```python
from build123d import *

# Parameters (mm, degrees)
F1_DEPTH = 15
F2_R     = 7.5
F3_DEPTH = 107.336067
F4_R     = 10
F5_DEPTH = 70


with BuildPart() as f1:
    # F0 (on Front) → F1 (new body, symmetric)
    with BuildSketch(Plane.XZ):
        with BuildLine():
            ThreePointArc((-30, 0), (-27.716386, 11.480503), (-21.213203, 21.213203))
            Line((-21.213203, 21.213203), (-70.710678, 70.710678))
            ThreePointArc((-70.710678, 70.710678), (-92.387953, 38.268343), (-100, 0))
            Line((-100, 0), (-30, 0))
        make_face()
        with BuildLine():
            ThreePointArc((-21.213203, -21.213203), (-27.716386, -11.480503), (-30, 0))
            Line((-30, 0), (-100, 0))
            ThreePointArc((-100, 0), (-92.387953, -38.268343), (-70.710678, -70.710678))
            Line((-70.710678, -70.710678), (-21.213203, -21.213203))
        make_face()
    extrude(amount=F1_DEPTH, both=True)

    # F2 (on Right) → F3 (cut)
    with BuildSketch(Plane.YZ):
        Circle(F2_R)
    extrude(amount=-F3_DEPTH, mode=Mode.SUBTRACT)

    # F4 (on Right) → F5 (cut)
    with BuildSketch(Plane.YZ):
        Circle(F4_R)
    extrude(amount=-F5_DEPTH, mode=Mode.SUBTRACT)


solid = f1.part
```
Geometry: final body of the model. Coordinates: model frame, mm. Round coordinates to 2 decimals unless told otherwise and drop trailing zeros. Loops run counter-clockwise (first coordinate to the right, second up) from the corner with the lowest first, then second, coordinate; pieces in that order, holes last.
Item 1: Mould query, pull axis Z, two halves, no side actions, for faces 1 (the cylindrical face through (-48.85, -2.17, -9.76)), 2 (the flat face through (-46, 0, 46)), 3 (the flat face through (-61, -15, 1)), 4 (the flat face through (-70, 4, 7)). Classes: released by +Z, released by -Z, zero draft, split by the parting line, or undercut.
Checked values:
face 1: undercut
face 2: released by +Z
face 3: zero draft
face 4: undercut
Item 2: Section D-D, the plane z = -60. Output: boundary loops of the cut face in (x, y).
Checked values:
outline: (-80, -15) - (-60, -15) - (-60, 15) - (-80, 15) - close
Item 3: Section C-C, the plane y = -12. Output: boundary loops of the cut face in (x, z).
Checked values:
outline: (-100, 0) arc R100 ccw to (-70.71, -70.71) - (-21.21, -21.21) arc R30 cw to (-30, 0) arc R30 cw to (-21.21, 21.21) - (-70.71, 70.71) arc R100 ccw to start
Item 4: Section B-B, the plane x = -73. Output: boundary loops of the cut face in (y, z).
Checked values:
outline: (-15, -68.34) - (15, -68.34) - (15, 68.34) - (-15, 68.34) - close; hole circle Ø15 at (0, 0)
Item 5: Contact query for flat-ended pins moving along their axis: P1, Ø12, axis at x = -90, y = -2.5, coming from the -Z side; P2, Ø1.5, axis at y = -5.5, z = 44.5, coming from the +X side; P3, Ø4, axis at x = -52, y = -11.5, coming from the -Z side. Output: stop coordinate, or through.
Checked values:
P1: stops at z = -54.26
P2: stops at x = -43.75
P3: stops at z = -54
Item 6: Section A-A, the plane y = 1. Output: boundary loops of the cut face in (x, z), plus the area to 3 significant figures.
Checked values:
outline: (-99.72, -7.43) arc R100 ccw to (-70.71, -70.71) - (-21.21, -21.21) arc R30 cw to (-28.3, -9.95) - (-70, -9.95) - (-70, -7.43) - close; (-99.72, 7.43) - (-70, 7.43) - (-70, 9.95) - (-28.3, 9.95) arc R30 cw to (-21.21, 21.21) - (-70.71, 70.71) arc R100 ccw to start
area: 5,900 mm2
Item 7: Line query: L1, parallel to Y at x = -75.5, z = 0; L2, parallel to Z at x = -79.5, y = -3; L3, parallel to Z at x = -64.5, y = -7.5. Output: solid intervals per line, ascending.
Checked values:
L1: y = -15 to -7.5, 7.5 to 15
L2: z = -60.66 to -6.87, 6.87 to 60.66
L3: z = -64.5 to -6.61, 6.61 to 64.5
